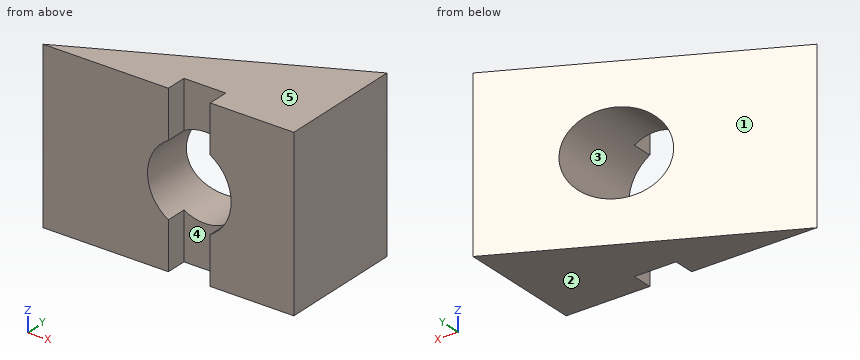
```python
from build123d import *

# Parameters (mm, degrees)
F1_DEPTH = 101.6
F3_W     = 25.4
F3_H     = 101.6
F4_DEPTH = 12.7
F5_R     = 25.4
F6_DEPTH = 76.201


with BuildPart() as f1:
    # F0 (on Top) → F1 (new body)
    with BuildSketch(Plane.XY):
        Polygon((152.4, 76.2), (0, 0), (152.4, 0), align=None)
    extrude(amount=F1_DEPTH)

    # F3 (on face) → F4 (cut)
    with BuildSketch(Plane.XZ):
        with Locations((88.9, 50.8)):
            Rectangle(F3_W, F3_H)
    extrude(amount=-F4_DEPTH, mode=Mode.SUBTRACT)

    # F5 (on face) → F6 (cut, through all)
    with BuildSketch(Plane.XZ):
        with Locations((88.907994, 50.733309)):
            Circle(F5_R)
    extrude(amount=-F6_DEPTH, mode=Mode.SUBTRACT)


solid = f1.part
```
Here's how the part is built. I have some questions about the finished solid (model axes, mm). Face numbers are marked on the shaded views. A direction names the side the tool comes from. Round coordinates to 2 decimals unless told otherwise and drop trailing zeros. Order: outer loops, then holes, each group sorted by start corner. A loop starts at its lowest first (then second) coordinate and runs counter-clockwise, first axis right, second up. Notation, with made-up numbers: (77.5, -14.5) -> (94.5, -14.5) arc R18 cw to (94.5, 20.5) -> close; hole circle Ø11 at (89, 53.5). An arc over 180 degrees is marked (long way). Use a Markdown table: item, result. Add a question column.
(1) For the marked faces 4 and 5, which set-ups out of +Z, -Z, +X, -X, +Y, -Y let a thin tool reach every point of the face, with its end or its side?
(2) I need wall thicknesses on line 1 along Z through (x, y) = (77.5, 26); line 2 along Z through (x, y) = (107.5, 51); line 3 along X through (y, z) = (12.5, 92). Which ranges of each line are inside material? Lowest first, please.
(3) Suppose I cut it at C-C, the plane y = 28.5. Please give me the cut outline in (x, z).
(4) Suppose I cut it at B-B, the plane x = 94. Please give me the cut outline in (y, z), and give its area (3 significant figures).
(5) If we mould it in two halves opening along X, with no side actions, what happens to the marked faces 1, 2 and 3? For each: released by +X, released by -X, zero draft, split by the parting line, or undercut.
(6) For pin 1 Ø12.5 at (x, z) = (92, 80.5) entering from -Y; pin 2 Ø3 at (y, z) = (67, 29.5) entering from -X; pin 3 Ø14 at (y, z) = (7.5, 11) entering from -X, each with a flat end and sliding along its axis, tell me the tip position at first contact or that it passes through.
(7) Suppose I cut it at A-A, the plane z = 32. Please give me the cut outline in (x, y).
(8) Suppose I cut it at D-D, the plane y = 70. Please give me the cut outline in (x, z).
Verdict:
| question | item | result |
|---|---|---|
| 1 | face 4 | +Z, -Z, -Y |
| 1 | face 5 | +Z, +X, -X, +Y, -Y |
| 2 | line 1 | 0 to 28.04, 73.43 to 101.6 |
| 2 | line 2 | 0 to 33.43, 68.04 to 101.6 |
| 2 | line 3 | 25 to 76.2, 101.6 to 152.4 |
| 3 | outline | (57, 0) -> (152.4, 0) -> (152.4, 101.6) -> (57, 101.6) -> close; hole circle Ø50.8 at (88.91, 50.73) |
| 4 | outline | (12.7, 0) -> (47, 0) -> (47, 25.85) -> (12.7, 25.85) -> close; (12.7, 75.62) -> (47, 75.62) -> (47, 101.6) -> (12.7, 101.6) -> close |
| 4 | area | 1,780 mm2 |
| 5 | face 1 | released by -X |
| 5 | face 2 | zero draft |
| 5 | face 3 | undercut |
| 6 | pin 1 | y = 12.7 |
| 6 | pin 2 | x = 131 |
| 6 | pin 3 | x = 1 |
| 7 | outline | (0, 0) -> (71.76, 0) -> (71.76, 35.88) -> close; (106.06, 0) -> (152.4, 0) -> (152.4, 76.2) -> (106.06, 53.03) -> close |
| 8 | outline | (140, 0) -> (152.4, 0) -> (152.4, 101.6) -> (140, 101.6) -> close |
